Could you check a few things on this model? Use its own coordinates, in mm. Face numbers are marked on the shaded views. Give positions to 0.01 mm unless a question says otherwise; leave off trailing zeros. Order: outer loops, then holes, each group sorted by start corner. A loop starts at its lowest first (then second) coordinate and runs counter-clockwise, first axis right, second up. Notation, with made-up numbers: M 72.25,80.5 L 99.25,80.5 A22 cw 99.25,114.5 Z; hole C 39,-19 d10. An arc over 180 degrees is marked long. Use a Markdown table: item, result. Add a question column.
Item 1: If we mould it in two halves opening along X, with no side actions, what happens to the marked faces 1, 2 and 3? For each: released by +X, released by -X, zero draft, split by the parting line, or undercut.
Item 2: Suppose I cut it at B-B on x = -32.5. Write out the boundary of the cut face in (y, z).
Item 3: I'm going to push a flat-ended pin straight in: pin 1 Ø2.5 at (x, y) = (-38, 47.01) entering from -Z. Where does the tip first touch, or does it pass through?
Item 4: Suppose I cut it at C-C on z = -9.75. Write out the boundary of the cut face in (x, y).
Item 5: If I drill on L1, parallel to X at y = 5.5, z = -1; L2, parallel to Y at x = 18, z = -4.5; L3, parallel to X at y = -8.5, z = -7.5, over which ranges is the centre line in solid material (lowest first)? Write a range as from..to.
Item 6: Suppose I cut it at A-A on y = -31. Write out the boundary of the cut face in (x, z), plus the area to 3 significant figures.
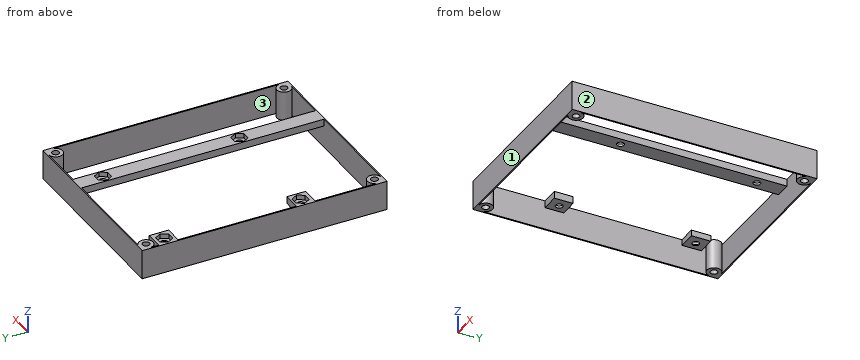
from build123d import *

# Parameters (mm, degrees)
SKETCH007_W     = 79.5
SKETCH007_H     = 104
SKETCH007_R     = 1.5
PAD002_DEPTH    = 12.5
SKETCH006_W     = 8.021301
SKETCH006_H     = 8.234894
SKETCH006_R     = 1.5
PAD001_DEPTH    = 2.5
POCKET005_DEPTH = 2
SKETCH033_W     = 7.946812
SKETCH033_H     = 7.946812
SKETCH033_R     = 1.5
PAD003_DEPTH    = 3
SKETCH034_W     = 6.801386
SKETCH034_H     = 103.670945
SKETCH034_R     = 1.5
PAD004_DEPTH    = 3
POCKET006_DEPTH = 2
POCKET007_DEPTH = 2
POCKET008_DEPTH = 2


with BuildPart() as part:
    # Sketch007 → Pad002 (new body)
    with BuildSketch(Plane.XY):
        with Locations((-2.25, 6.5)):
            Rectangle(SKETCH007_W, SKETCH007_H)
        with Locations((-38.5, 55)):
            Circle(SKETCH007_R, mode=Mode.SUBTRACT)
        with Locations((34, 55)):
            Circle(SKETCH007_R, mode=Mode.SUBTRACT)
        with Locations((-38.5, -42)):
            Circle(SKETCH007_R, mode=Mode.SUBTRACT)
        with Locations((34, -42)):
            Circle(SKETCH007_R, mode=Mode.SUBTRACT)
        with BuildLine():
            Line((34, -45), (-38.5, -45))
            ThreePointArc((-38.5, -45), (-36.37868, -39.87868), (-41.5, -42))
            Line((-41.5, -42), (-41.5, 55))
            ThreePointArc((-41.5, 55), (-36.37868, 52.87868), (-38.5, 58))
            Line((-38.5, 58), (34, 58))
            ThreePointArc((34, 58), (31.87868, 52.87868), (37, 55))
            Line((37, 55), (37, -42))
            ThreePointArc((37, -42), (31.87868, -39.87868), (34, -45))
        make_face(mode=Mode.SUBTRACT)
    extrude(amount=-PAD002_DEPTH)

    # Sketch006 → Pad001 (join)
    with BuildSketch(Plane.XY):
        with Locations((-37.87762, 47.077984)):
            Rectangle(SKETCH006_W, SKETCH006_H)
        with Locations((-37.997646, 47.010536)):
            Circle(SKETCH006_R, mode=Mode.SUBTRACT)
    extrude(amount=-PAD001_DEPTH)

    # Sketch032 (on Face23 of Pad001) → Pocket005 (cut)
    with BuildSketch(Plane.XY):
        Polygon((-34.726036, 46.982567), (-36.351036, 49.79715), (-39.601036, 49.79715), (-41.226036, 46.982567), (-39.601036, 44.167984), (-36.351036, 44.167984), align=None)
    extrude(amount=-POCKET005_DEPTH, mode=Mode.SUBTRACT)

    # Sketch033 → Pad003 (join)
    with BuildSketch(Plane.XY):
        with Locations((-37.923063, -11.232048)):
            Rectangle(SKETCH033_W, SKETCH033_H)
        with Locations((-37.99107, -11.008605)):
            Circle(SKETCH033_R, mode=Mode.SUBTRACT)
    extrude(amount=-PAD003_DEPTH)

    # Sketch034 → Pad004 (join)
    with BuildSketch(Plane.XY):
        with Locations((10.981288, 6.512218)):
            Rectangle(SKETCH034_W, SKETCH034_H)
        with Locations((11.033937, 47.026531)):
            Circle(SKETCH034_R, mode=Mode.SUBTRACT)
        with Locations((11.033937, -10.967275)):
            Circle(SKETCH034_R, mode=Mode.SUBTRACT)
    extrude(amount=-PAD004_DEPTH)

    # Sketch035 (on Face34 of Pad004) → Pocket006 (cut)
    with BuildSketch(Plane.XY):
        Polygon((-36.326836, -8.14599), (-39.576836, -8.14599), (-41.201836, -10.960573), (-39.576836, -13.775156), (-36.326836, -13.775156), (-34.701836, -10.960573), align=None)
    extrude(amount=-POCKET006_DEPTH, mode=Mode.SUBTRACT)

    # Sketch036 (on Face26 of Pocket006) → Pocket007 (cut)
    with BuildSketch(Plane.XY):
        Polygon((12.678073, 49.85376), (9.428073, 49.85376), (7.803073, 47.039177), (9.428073, 44.224594), (12.678073, 44.224594), (14.303073, 47.039177), align=None)
    extrude(amount=-POCKET007_DEPTH, mode=Mode.SUBTRACT)

    # Sketch037 (on Face26 of Pocket007) → Pocket008 (cut)
    with BuildSketch(Plane.XY):
        Polygon((12.636199, -8.121596), (9.386199, -8.121596), (7.761199, -10.936179), (9.386199, -13.750762), (12.636199, -13.750762), (14.261199, -10.936179), align=None)
    extrude(amount=-POCKET008_DEPTH, mode=Mode.SUBTRACT)


solid = part.part
Findings below:
| question | item | result |
|---|---|---|
| 1 | face 1 | zero draft |
| 1 | face 2 | released by +X |
| 1 | face 3 | undercut |
| 2 | outline | M -45.5,-12.5 L -45,-12.5 L -45,0 L -45.5,0 Z; M 58,-12.5 L 58.5,-12.5 L 58.5,0 L 58,0 Z |
| 3 | pin 1 | passes through |
| 4 | outline | M -42,-45.5 L 37.5,-45.5 L 37.5,58.5 L -42,58.5 Z; hole M -41.5,-42 A3 cw long -38.5,-45 L 34,-45 A3 cw long 37,-42 L 37,55 A3 cw long 34,58 L -38.5,58 A3 cw long -41.5,55 Z; hole C -38.5,-42 d3; hole C -38.5,55 d3; hole C 34,-42 d3; hole C 34,55 d3 |
| 5 | L1 | x = -42..-41.5, 7.58..14.38, 37..37.5 |
| 5 | L2 | y = -45.5..-45, 58..58.5 |
| 5 | L3 | x = -42..-41.5, 37..37.5 |
| 6 | outline | M -42,-12.5 L -41.5,-12.5 L -41.5,0 L -42,0 Z; M 7.58,-3 L 14.38,-3 L 14.38,0 L 7.58,0 Z; M 37,-12.5 L 37.5,-12.5 L 37.5,0 L 37,0 Z |
| 6 | area | 32.9 mm^2 |
